Here's how the part is built. I have some questions about the finished solid (model axes, mm). Face numbers are marked on the shaded views. Round coordinates to 2 decimals unless told otherwise and drop trailing zeros. Loops run counter-clockwise (first coordinate to the right, second up) from the corner with the lowest first, then second, coordinate; pieces in that order, holes last. Notation, with made-up numbers: (20.5, 87.5) -> (56.5, 87.5) arc R20 cw to (56.5, 121.5) -> close; hole circle Ø3 at (40, -30). An arc over 180 degrees is marked (long way). Use one line per item in the form item = value. Start each with the question number.
Item 1: I'm going to push flat-ended pins straight in: pin 1 Ø1.5 at (y, z) = (-27.5, 4) entering from +X; pin 2 Ø1.5 at (x, z) = (-41.5, 4) entering from +Y; pin 3 Ø5 at (y, z) = (0, 16.5) entering from -X. Where does each tip first touch, or does it pass through?
Item 2: If we section it at A-A (y = -8.5): Write out the boundary of the cut face in (x, z), then the cut area to 3 significant figures.
Item 3: If we section it at C-C (z = 5.25): State how many separate pieces and enclosed holes the cut face has, then the cut area to 3 significant figures.
Item 4: If we section it at D-D (y = 47): Write out the boundary of the cut face in (x, z).
Item 5: If I drill on L1, parallel to Y at x = 0, z = 8.25; L2, parallel to X at y = -2.5, z = 5.25; L3, parallel to X at y = -1, z = 14.25, over which ranges is the centre line in solid material (lowest first)? Write a range as [from, to].
Item 6: If we section it at B-B (x = 38.1): Write out the boundary of the cut face in (y, z).
Item 7: Thinking about a two-plate mould opening in Y: for the marked faces 1, 2, 3 and 4, which applies, released by +Y, released by -Y, zero draft, split by the parting line, or undercut?
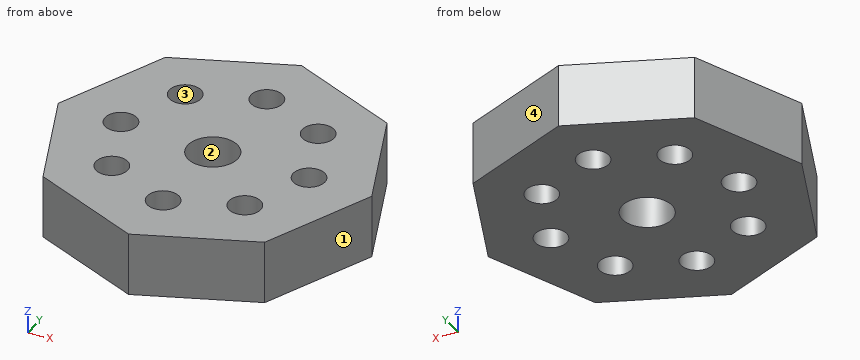
```python
from build123d import *

# Parameters (mm, degrees)
F0_R     = 6.35
F1_DEPTH = 25.4
F2_R     = 9.978597
F3_DEPTH = 25.4


with BuildPart() as f1:
    # F0 (on Top) → F1 (new body)
    with BuildSketch(Plane.XY):
        Polygon((44.901281, -44.901281), (63.5, 0), (44.901281, 44.901281), (0, 63.5), (-44.901281, 44.901281), (-63.5, 0), (-44.901281, -44.901281), (0, -63.5), align=None)
        with Locations((-26.940768, -26.940768)):
            Circle(F0_R, mode=Mode.SUBTRACT)
        with Locations((0, -38.1)):
            Circle(F0_R, mode=Mode.SUBTRACT)
        with Locations((26.940768, -26.940768)):
            Circle(F0_R, mode=Mode.SUBTRACT)
        with Locations((-38.1, 0)):
            Circle(F0_R, mode=Mode.SUBTRACT)
        with Locations((-26.940768, 26.940768)):
            Circle(F0_R, mode=Mode.SUBTRACT)
        with Locations((26.940768, 26.940768)):
            Circle(F0_R, mode=Mode.SUBTRACT)
        with Locations((38.1, 0)):
            Circle(F0_R, mode=Mode.SUBTRACT)
        with Locations((0, 38.1)):
            Circle(F0_R, mode=Mode.SUBTRACT)
    extrude(amount=F1_DEPTH)

    # F2 (on face) → F3 (cut)
    with BuildSketch(Plane.XY.offset(25.4)):
        with Locations((0, -1.644041)):
            Circle(F2_R)
    extrude(amount=-F3_DEPTH, mode=Mode.SUBTRACT)


solid = f1.part
```
Values found:
q1.pin_1 = 52.42
q1.pin_2 = 46.62
q1.pin_3 = -63.5
q2.outline = (-59.98, 0) -> (-7.25, 0) -> (-7.25, 25.4) -> (-59.98, 25.4) -> close; (7.25, 0) -> (59.98, 0) -> (59.98, 25.4) -> (7.25, 25.4) -> close
q2.area = 2,680 mm2
q3.separate_pieces = 1
q3.enclosed_holes = 9
q3.area = 10,100 mm2
q4.outline = (-39.83, 0) -> (39.83, 0) -> (39.83, 25.4) -> (-39.83, 25.4) -> close
q5.L1 = [-63.5, -44.45], [-31.75, -11.62], [8.33, 31.75], [44.45, 63.5]
q5.L2 = [-62.46, -43.94], [-32.26, -9.94], [9.94, 32.26], [43.94, 62.46]
q5.L3 = [-63.09, -44.37], [-31.83, -9.96], [9.96, 31.83], [44.37, 63.09]
q6.outline = (-47.72, 0) -> (-6.35, 0) -> (-6.35, 25.4) -> (-47.72, 25.4) -> close; (6.35, 0) -> (47.72, 0) -> (47.72, 25.4) -> (6.35, 25.4) -> close
q7.face_1 = released by -Y
q7.face_2 = undercut
q7.face_3 = undercut
q7.face_4 = released by +Y
